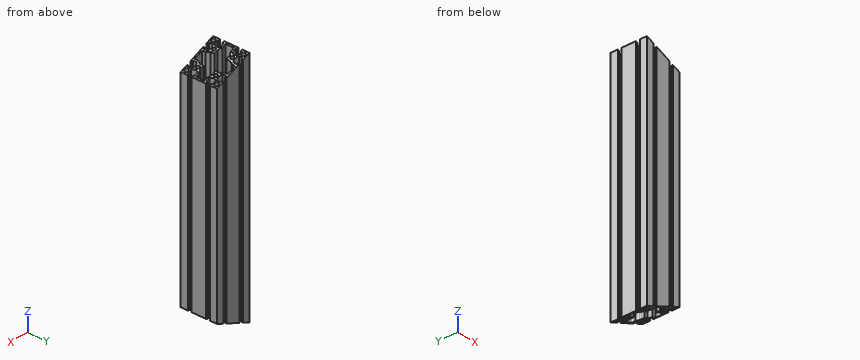
from build123d import *

# Parameters (mm, degrees)
F0_R          = 3
F0_R_2        = 2.5
F1_DEPTH      = 389.7
F2_R          = 2
F3_R          = 7
F5_DEPTH      = 30
F5_DEPTH_BACK = 30


# Not quite as in the source:
# - a feature names something its author has since deleted; it is built from what else it names


with BuildPart() as f1:
    # F0 (on Top) → F1 (new body)
    with BuildSketch(Plane.XY):
        with BuildLine():
            Line((18.15, -30), (30, -30))
            Line((30, -30), (30, -18.15))
            Line((30, -18.15), (27.5, -18.15))
            Line((27.5, -18.15), (27.5, -20.15))
            Line((27.5, -20.15), (21.5477069044, -20.15))
            ThreePointArc((21.5477069044, -20.15), (19.5, -15), (21.5477069044, -9.85))
            Line((21.5477069044, -9.85), (27.5, -9.85))
            Line((27.5, -9.85), (27.5, -11.85))
            Line((27.5, -11.85), (30, -11.85))
            Line((30, -11.85), (30, 11.85))
            Line((30, 11.85), (27.5, 11.85))
            Line((27.5, 11.85), (27.5, 9.85))
            Line((27.5, 9.85), (21.5477069044, 9.85))
            ThreePointArc((21.5477069044, 9.85), (19.5, 15), (21.5477069044, 20.15))
            Line((21.5477069044, 20.15), (27.5, 20.15))
            Line((27.5, 20.15), (27.5, 18.15))
            Line((27.5, 18.15), (30, 18.15))
            Line((30, 18.15), (30, 30))
            Line((30, 30), (18.15, 30))
            Line((18.15, 30), (18.15, 27.5))
            Line((18.15, 27.5), (20.15, 27.5))
            Line((20.15, 27.5), (20.15, 21.5477069044))
            ThreePointArc((20.15, 21.5477069044), (15, 19.5), (9.85, 21.5477069044))
            Line((9.85, 21.5477069044), (9.85, 27.5))
            Line((9.85, 27.5), (11.85, 27.5))
            Line((11.85, 27.5), (11.85, 30))
            Line((11.85, 30), (-11.85, 30))
            Line((-11.85, 30), (-11.85, 27.5))
            Line((-11.85, 27.5), (-9.85, 27.5))
            Line((-9.85, 27.5), (-9.85, 21.5477069044))
            ThreePointArc((-9.85, 21.5477069044), (-15, 19.5), (-20.15, 21.5477069044))
            Line((-20.15, 21.5477069044), (-20.15, 27.5))
            Line((-20.15, 27.5), (-18.15, 27.5))
            Line((-18.15, 27.5), (-18.15, 30))
            Line((-18.15, 30), (-30, 30))
            Line((-30, 30), (-30, 18.15))
            Line((-30, 18.15), (-27.5, 18.15))
            Line((-27.5, 18.15), (-27.5, 20.15))
            Line((-27.5, 20.15), (-21.5477069044, 20.15))
            ThreePointArc((-21.5477069044, 20.15), (-19.5, 15), (-21.5477069044, 9.85))
            Line((-21.5477069044, 9.85), (-27.5, 9.85))
            Line((-27.5, 9.85), (-27.5, 11.85))
            Line((-27.5, 11.85), (-30, 11.85))
            Line((-30, 11.85), (-30, -11.85))
            Line((-30, -11.85), (-27.5, -11.85))
            Line((-27.5, -11.85), (-27.5, -9.85))
            Line((-27.5, -9.85), (-21.5477069044, -9.85))
            ThreePointArc((-21.5477069044, -9.85), (-19.5, -15), (-21.5477069044, -20.15))
            Line((-21.5477069044, -20.15), (-27.5, -20.15))
            Line((-27.5, -20.15), (-27.5, -18.15))
            Line((-27.5, -18.15), (-30, -18.15))
            Line((-30, -18.15), (-30, -30))
            Line((-30, -30), (-18.15, -30))
            Line((-18.15, -30), (-18.15, -27.5))
            Line((-18.15, -27.5), (-20.15, -27.5))
            Line((-20.15, -27.5), (-20.15, -21.5477069044))
            ThreePointArc((-20.15, -21.5477069044), (-15, -19.5), (-9.85, -21.5477069044))
            Line((-9.85, -21.5477069044), (-9.85, -27.5))
            Line((-9.85, -27.5), (-11.85, -27.5))
            Line((-11.85, -27.5), (-11.85, -30))
            Line((-11.85, -30), (11.85, -30))
            Line((11.85, -30), (11.85, -27.5))
            Line((11.85, -27.5), (9.85, -27.5))
            Line((9.85, -27.5), (9.85, -21.5477069044))
            ThreePointArc((9.85, -21.5477069044), (15, -19.5), (20.15, -21.5477069044))
            Line((20.15, -21.5477069044), (20.15, -27.5))
            Line((20.15, -27.5), (18.15, -27.5))
            Line((18.15, -27.5), (18.15, -30))
        make_face()
        with Locations((-25, -25)):
            Circle(F0_R, mode=Mode.SUBTRACT)
        with Locations((-15, -15)):
            Circle(F0_R_2, mode=Mode.SUBTRACT)
        with Locations((25, -25)):
            Circle(F0_R, mode=Mode.SUBTRACT)
        with Locations((15, -15)):
            Circle(F0_R_2, mode=Mode.SUBTRACT)
        with Locations((-25, 25)):
            Circle(F0_R, mode=Mode.SUBTRACT)
        with Locations((-15, 15)):
            Circle(F0_R_2, mode=Mode.SUBTRACT)
        Polygon((-7, 22), (-7, 27.5), (0, 27.5), (7, 27.5), (7, 22), (10, 16), (10, 10), (16, 10), (22, 7), (27.5, 7), (27.5, 0), (27.5, -7), (22, -7), (16, -10), (10, -10), (10, -16), (7, -22), (7, -27.5), (0, -27.5), (-7, -27.5), (-7, -22), (-10, -16), (-10, -10), (-16, -10), (-22, -7), (-27.5, -7), (-27.5, 0), (-27.5, 7), (-22, 7), (-16, 10), (-10, 10), (-10, 16), align=None, mode=Mode.SUBTRACT)
        with Locations((15, 15)):
            Circle(F0_R_2, mode=Mode.SUBTRACT)
        with Locations((25, 25)):
            Circle(F0_R, mode=Mode.SUBTRACT)
    extrude(amount=F1_DEPTH)

    # F2
    f2_edges = [f1.edges().sort_by_distance(p)[0] for p in [
        (-7, 27.5, 194.85),
        (7, 27.5, 194.85),
    ]]
    fillet(f2_edges, radius=F2_R)

    # F3
    f3_edges = [f1.edges().sort_by_distance(p)[0] for p in [
        (-10, 16, 194.85),
        (10, 16, 194.85),
    ]]
    fillet(f3_edges, radius=F3_R)

    # F4 (on Front) → F5 (cut, two sides)
    with BuildSketch(Plane.XZ) as f5_sk:
        Polygon((262.6101504464, 391.20035759), (13.3822209239, 494.4339461204), (-30, 389.7), (219.2279295224, 286.4664114696), align=None)
        Polygon((237.6533260841, 110.8656376783), (-30, 0), (20.6125739706, -122.1895625065), (288.2659000547, -11.3239248282), align=None)
    extrude(amount=F5_DEPTH, mode=Mode.SUBTRACT)
    extrude(f5_sk.sketch, amount=-F5_DEPTH_BACK, mode=Mode.SUBTRACT)


solid = f1.part
Verification items for the finished model (mm, model axes). Coordinates: 2 decimals unless noted, no trailing zeros. Order: outer loops, then holes, each group sorted by start corner. A loop starts at its lowest first (then second) coordinate and runs counter-clockwise, first axis right, second up.
1. Sectioned sample at A-A, the plane x = 0. Record the cut outline in (y, z), and give its area (3 significant figures).
Results found:
outline: (-30, 12.43) - (-27.5, 12.43) - (-27.5, 377.27) - (-30, 377.27) - close; (27.5, 12.43) - (30, 12.43) - (30, 377.27) - (27.5, 377.27) - close
area: 1,820 mm2
2. Go/stop test with flat-tipped pins: pin 1 Ø5 at (x, z) = (13, 208) entering from +Y; pin 2 Ø10 at (x, y) = (-14, -14) entering from -Z; pin 3 Ø4 at (x, y) = (15, -15) entering from +Z. Record where each tip stops, or that it passes through.
Results found:
pin 1: stops at y = 30
pin 2: stops at z = 4.56
pin 3: passes through
3. Sectioned sample at B-B, the plane z = 106.5. Give the number of separate pieces and of enclosed holes in the cut face, and give its area (3 significant figures).
Results found:
separate pieces: 1
enclosed holes: 9
area: 1,080 mm2
4. Scan lines: line 1 (X direction, y = 25, z = 200); line 2 (X direction, y = -15, z = 268). Record each from-to range of solid material in increasing order.
Results found:
line 1: x = -30 to -28, -22 to -20.15, -9.85 to -7, 7 to 9.85, 20.15 to 22, 28 to 30
line 2: x = -19.5 to -17.5, -12.5 to -10, 10 to 12.5, 17.5 to 19.5
